from build123d import *

# Parameters (mm, degrees)
SKETCH5_R      = 1.397
SKETCH5_R_2    = 1.362219034
EXTRUDE1_DEPTH = 2.286


with BuildPart() as part:
    # Sketch5 → Extrude1 (new body)
    with BuildSketch(Plane(origin=(0, 0, 0), x_dir=(-0.018375543, 0.999831155, 0), z_dir=(0, 0, -1))):
        with BuildLine():
            Line((33.80665155, 26.18621859), (34.46394605, -9.577814671))
            ThreePointArc((34.46394605, -9.577814671), (31.404055355, -10.348947358), (28.630167887, -11.853315998))
            Line((28.630167887, -11.853315998), (23.830153765, -23.292701447))
            Line((23.830153765, -23.292701447), (8.486225874, -20.477486777))
            ThreePointArc((8.486225874, -20.477486777), (-7.865336256, 12.262044577), (24.425706506, 29.482353943))
            Line((24.425706506, 29.482353943), (33.80665155, 26.18621859))
        make_face()
        with Locations((27.527734531, 22.260177192)):
            Circle(SKETCH5_R, mode=Mode.SUBTRACT)
        with Locations((30.179746314, -4.890797216)):
            Circle(SKETCH5_R, mode=Mode.SUBTRACT)
        with Locations((3.363138785, 18.996048152)):
            Circle(SKETCH5_R_2, mode=Mode.SUBTRACT)
        with Locations((0.317842079, -7.407837933)):
            Circle(SKETCH5_R, mode=Mode.SUBTRACT)
    extrude(amount=EXTRUDE1_DEPTH)


solid = part.part
Model file for the job. Use its own axes, mm. Give positions to 0.01 mm unless a question says otherwise; leave off trailing zeros. Order: outer loops, then holes, each group sorted by start corner. A loop starts at its lowest first (then second) coordinate and runs counter-clockwise, first axis right, second up. Notation, with made-up numbers: M 59.5,78.25 L 70.5,78.25 A10 cw 70.5,83.25 Z; hole C 42,-34 d1. An arc over 180 degrees is marked long. Put each result on its own line as item: value. Start each with the question number.
(1) Band-saw the part on B-B on x = -16.5. Give the cut face in (y, z), then the cut area to 3 significant figures.
(2) Drill centre lines: L1, parallel to Y at x = 4, z = -0.3; L2, parallel to Y at x = 0.5, z = -1.75; L3, parallel to X at y = 29.5, z = -0.95. Where is each one in solid material? Low to high. Write a range as [from, to].
(3) Band-saw the part on A-A on z = -0.45. Give the cut face in (x, y).
(4) Pull direction Y, two halves, no side cores. Call faces 1 (the face through (27.32, 29.56, -1.13)), 2 (the face through (4, 13, 0)), 3 (the face through (-5.049, 31.425, -1.127)), 4 (the face through (17.607, 3.392, -1.127)): released by +Y, released by -Y, zero draft, split by the parting line, or undercut.
(5) Pin check, flat tips, straight feed: pin 1 Ø1.5 at (x, y) = (-9, 6.5) entering from +Z; pin 2 Ø1.7 at (x, y) = (-5.44, 30.08) entering from -Z. Stop position of each tip, or through.
(6) Band-saw the part on C-C on y = 13.5. Give the cut face in (x, z), then the cut area to 3 significant figures.
Results below:
1. outline: M 0.8,-2.29 L 26.59,-2.29 L 26.59,0 L 0.8,0 Z
1. area: 58.9 mm2
2. L1: y = [-9.03, 34.28]
2. L2: y = [-8.8, 34.28]
2. L3: x = [-11.7, -6.71], [-4.18, 27.34]
3. outline: M -23.73,23.4 L -20.63,8.11 A26.23 ccw 29.03,24.96 L 25.56,34.28 L -10.21,34.28 A12.65 cw -12.38,28.41 Z; hole C -7.41,0.18 d2.79; hole C -5.44,30.08 d2.79; hole C 18.93,3.71 d2.72; hole C 21.75,27.93 d2.79
4. face 1: released by +Y
4. face 2: zero draft
4. face 3: undercut
4. face 4: undercut
5. pin 1: stops at z = 0
5. pin 2: passes through
6. outline: M -21.72,-2.29 L 29.94,-2.29 L 29.94,0 L -21.72,0 Z
6. area: 118 mm2
